Drawing for the job (mm, zero at the part's lowest x, y, z). A direction names the side the tool comes from. Coordinates: 2 decimals unless noted, no trailing zeros. Loops run counter-clockwise (first coordinate to the right, second up) from the corner with the lowest first, then second, coordinate; pieces in that order, holes last. Notation, with made-up numbers: (13, -26.5) -> (62, -26.5) arc R29 ccw to (62, 5.5) -> close; hole circle Ø3 at (41.5, 34). An arc over 180 degrees is marked (long way). Write each question's results on one line, items separated by ' | '.
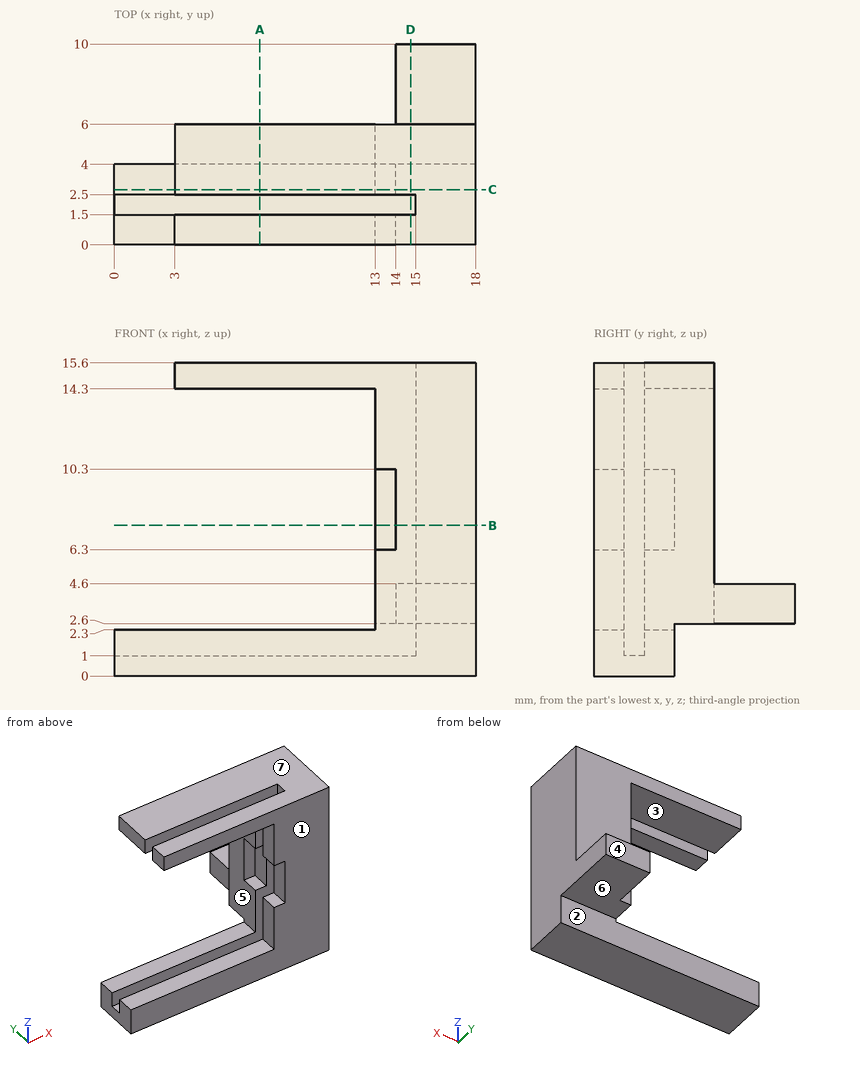
1) Pin check, flat tips, straight feed: pin 1 (4 mm diameter, centred on x = 16.5, y = 7.5, fed in from -Z); pin 2 (3 mm diameter, centred on x = 9.5, z = 11, fed in from -Y); pin 3 (0.8 mm diameter, centred on x = 13.5, z = 9.5, fed in from -Y); pin 4 (2 mm diameter, centred on y = 4, z = 9, fed in from -X). Stop position of each tip, or through.
Outcome:
pin 1: stops at z = 2.6 | pin 2: passes through | pin 3: stops at y = 4 | pin 4: stops at x = 13
2) Which spindle directions (+Z, -Z, +X, -X, +Y, -Y) get a long thin tool onto all of the face, cutting with end or side? Do the marked faces 1, 2 and 3. Say none if no direction does.
Outcome:
face 1: +Z, -Z, +X, -X, -Y | face 2: -Z, +X, -X, +Y | face 3: -X, +Y, -Y
3) Slice it at A-A (x = 7.25). Write the cut outline in (y, z).
Outcome:
outline: (0, 0) -> (4, 0) -> (4, 2.3) -> (2.5, 2.3) -> (2.5, 1) -> (1.5, 1) -> (1.5, 2.3) -> (0, 2.3) -> close; (0, 14.3) -> (1.5, 14.3) -> (1.5, 15.6) -> (0, 15.6) -> close; (2.5, 14.3) -> (6, 14.3) -> (6, 15.6) -> (2.5, 15.6) -> close
4) Slice it at B-B (z = 7.5). Write the cut outline in (x, y).
Outcome:
outline: (13, 4) -> (14, 4) -> (14, 2.5) -> (15, 2.5) -> (15, 1.5) -> (14, 1.5) -> (14, 0) -> (18, 0) -> (18, 6) -> (13, 6) -> close
5) Two-plate mould, pull along Z, no slides. Class the marked faces 4, 5, 6 and 7: pulls with the +Z half, pulls with the -Z half, needs draft (parallel to the pull), parting line crosses it, or undercut.
Outcome:
face 4: needs draft | face 5: undercut | face 6: pulls with the -Z half | face 7: pulls with the +Z half
6) Drill centre lines: L1, parallel to Z at x = 5.5, y = 3.75; L2, parallel to Y at x = 11, z = 15.25; L3, parallel to Y at x = 15.5, z = 12.25. Where is each one in solid material? Low to high. Write a range as from..to.
Outcome:
L1: z = 0..2.3, 14.3..15.6 | L2: y = 0..1.5, 2.5..6 | L3: y = 0..6
7) Slice it at D-D (x = 14.75). Write the cut outline in (y, z), then the cut area to 3 significant figures.
Outcome:
outline: (0, 0) -> (4, 0) -> (4, 2.6) -> (10, 2.6) -> (10, 4.6) -> (6, 4.6) -> (6, 15.6) -> (2.5, 15.6) -> (2.5, 1) -> (1.5, 1) -> (1.5, 15.6) -> (0, 15.6) -> close | area: 81.8 mm^2
8) Slice it at C-C (y = 2.75). Write the cut outline in (x, z).
Outcome:
outline: (0, 0) -> (18, 0) -> (18, 15.6) -> (3, 15.6) -> (3, 14.3) -> (13, 14.3) -> (13, 10.3) -> (14, 10.3) -> (14, 6.3) -> (13, 6.3) -> (13, 2.3) -> (0, 2.3) -> close
